The model under review builds one solid part; all positions refer to its coordinate system, in mm. Coordinates: 2 decimals unless noted, no trailing zeros. Write each loop counter-clockwise with the first axis right and the second up, starting at its lowest first coordinate (ties: lowest second). Pieces come first, ordered by that corner, then holes.
1) Add section C-C, the plane z = 0.75. Give the number of separate pieces and of enclosed holes in the cut face, then the cut area to 3 significant figures.
2) Add section D-D, the plane x = -34.5. State the section outline as (y, z) points, then the cut area to 3 significant figures.
3) For P1, Ø1.5, axis at y = 16.5, z = 3.5, coming from the +X side; P2, Ø8, axis at x = -13, y = -3.5, coming from the -Z side; P3, Ø6.5, axis at x = 40, y = 0, coming from the -Z side; P4, Ø1.6, axis at x = -71.5, z = 1.5, coming from the +Y side, all flat-tipped, find the tip position at first contact; note any pin that passes through.
4) Add section B-B, the plane x = 40. State the section outline as (y, z) points, then the cut area to 3 significant figures.
5) For line 1 (X direction, y = 14.5, z = 2.1); line 2 (X direction, y = 11.5, z = 2.1); line 3 (Y direction, x = 40, z = 1.2), list the stretches that pass through material, from the lowest coordinate up.
6) Add section A-A, the plane y = 8.5. State the section outline as (x, z) points.
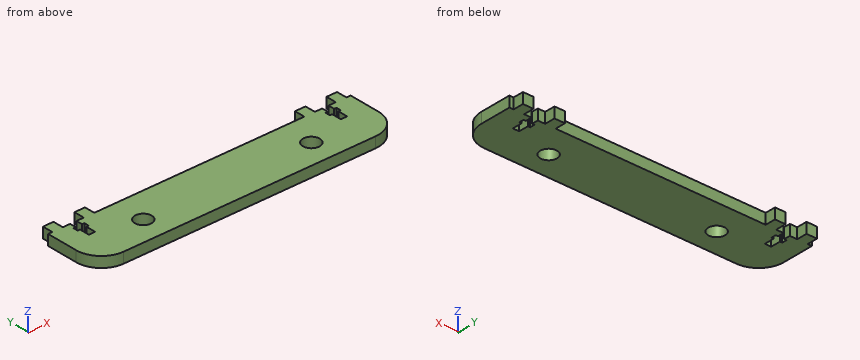
from build123d import *

# Parameters (mm, degrees)
SKETCH1_R           = 4
SKETCH1_W           = 5
SKETCH1_H           = 5
BOSS_EXTRUDE2_DEPTH = 5


with BuildPart() as part:
    # Sketch1 → Boss-Extrude2 (new body)
    # profile 1 of 5: a face of its own
    with BuildSketch(Plane.XY):
        with BuildLine():
            Line((-72, 15), (-72, 0))
            ThreePointArc((-72, 0), (-68.485281374, -8.485281374), (-60, -12))
            Line((-60, -12), (60, -12))
            ThreePointArc((60, -12), (68.485281374, -8.485281374), (72, 0))
            Line((72, 0), (72, 15))
            Line((72, 15), (70, 15))
            Line((70, 15), (65, 15))
            Line((65, 15), (61.5, 15))
            Line((61.5, 15), (61.5, 12))
            Line((61.5, 12), (62.6, 12))
            Line((62.6, 12), (62.6, 9.7))
            Line((62.6, 9.7), (61.5, 9.7))
            Line((61.5, 9.7), (61.5, 5))
            Line((61.5, 5), (58.5, 5))
            Line((58.5, 5), (58.5, 9.7))
            Line((58.5, 9.7), (57.4, 9.7))
            Line((57.4, 9.7), (57.4, 12))
            Line((57.4, 12), (58.5, 12))
            Line((58.5, 12), (58.5, 15))
            Line((58.5, 15), (55, 15))
            Line((55, 15), (50, 15))
            Line((50, 15), (-50, 15))
            Line((-50, 15), (-55, 15))
            Line((-55, 15), (-58.5, 15))
            Line((-58.5, 15), (-58.5, 12))
            Line((-58.5, 12), (-57.4, 12))
            Line((-57.4, 12), (-57.4, 9.7))
            Line((-57.4, 9.7), (-58.5, 9.7))
            Line((-58.5, 9.7), (-58.5, 5))
            Line((-58.5, 5), (-61.5, 5))
            Line((-61.5, 5), (-61.5, 9.7))
            Line((-61.5, 9.7), (-62.6, 9.7))
            Line((-62.6, 9.7), (-62.6, 12))
            Line((-62.6, 12), (-61.5, 12))
            Line((-61.5, 12), (-61.5, 15))
            Line((-61.5, 15), (-65, 15))
            Line((-65, 15), (-70, 15))
            Line((-70, 15), (-72, 15))
        make_face()
        with Locations((-40, 0)):
            Circle(SKETCH1_R, mode=Mode.SUBTRACT)
        with Locations((40, 0)):
            Circle(SKETCH1_R, mode=Mode.SUBTRACT)
    # profile 2 of 5: a face of its own
    with BuildSketch(Plane.XY):
        with Locations((52.5, 17.5)):
            Rectangle(SKETCH1_W, SKETCH1_H)
    # profile 3 of 5: a face of its own
    with BuildSketch(Plane.XY):
        with Locations((67.5, 17.5)):
            Rectangle(SKETCH1_W, SKETCH1_H)
    # profile 4 of 5: a face of its own
    with BuildSketch(Plane.XY):
        with Locations((-67.5, 17.5)):
            Rectangle(SKETCH1_W, SKETCH1_H)
    # profile 5 of 5: a face of its own
    with BuildSketch(Plane.XY):
        with Locations((-52.5, 17.5)):
            Rectangle(SKETCH1_W, SKETCH1_H)
    extrude(amount=BOSS_EXTRUDE2_DEPTH)


solid = part.part
Geometry results:
1. separate pieces: 1
1. enclosed holes: 2
1. area: 3,760 mm2
2. outline: (-12, 0) - (15, 0) - (15, 5) - (-12, 5) - close
2. area: 135 mm2
3. P1: stops at x = 70
3. P2: stops at z = 0
3. P3: passes through
3. P4: stops at y = 15
4. outline: (-12, 0) - (-4, 0) - (-4, 5) - (-12, 5) - close; (4, 0) - (15, 0) - (15, 5) - (4, 5) - close
4. area: 95.0 mm2
5. line 1: x = -72 to -61.5, -58.5 to 58.5, 61.5 to 72
5. line 2: x = -72 to -62.6, -57.4 to 57.4, 62.6 to 72
5. line 3: y = -12 to -4, 4 to 15
6. outline: (-72, 0) - (-61.5, 0) - (-61.5, 5) - (-72, 5) - close; (-58.5, 0) - (58.5, 0) - (58.5, 5) - (-58.5, 5) - close; (61.5, 0) - (72, 0) - (72, 5) - (61.5, 5) - close
